Autodesk Inventor part; units mm, degrees
ref_plane "YZ Plane" through (0, 0, 0) normal (1, 0, 0) x (0, 1, 0)
ref_plane "XZ Plane" through (0, 0, 0) normal (0, 1, 0) x (-1, 0, 0)
ref_plane "XY Plane" through (0, 0, 0) normal (0, 0, 1) x (1, 0, 0)
sketch "Эскиз1" plane through (0, 0, 0) normal (0, 0, 1) x (1, 0, 0)
  line L0 (-90.9717, -10.4774) -> (94.0283, -10.4774)
  line L1 (94.0283, -10.4774) -> (94.0283, 19.5226)
  line L2 (94.0283, 19.5226) -> (-90.9717, 19.5226)
  line L3 (-90.9717, 19.5226) -> (-90.9717, -10.4774)
  dimension "d2" = 185
  dimension "parametr_D" = 30
extrude "Выдавливание1" add sketch "Эскиз1" along normal blind 180
fillet "Сопряжение1" radius 42 1 edges at (94.0283, 4.5226, 180)
sketch "Эскиз3" plane through (-90.9717, -10.4774, 0) normal (0, -1, 0) x (1, 0, 0)
  point P0 (115, 21.3555)
sketch "Эскиз4" plane through (-90.9717, -10.4774, 0) normal (0, -1, 0) x (1, 0, 0)
  point P0 (15, 33)
equation "\"d2\" = parametr_A_"
equation "\"parametr_D\" = parametr_C_"
equation "\"d4\" = parametr_B_"
properties part number "lw_6_part2"
The model under review builds one solid part; all positions refer to its coordinate system, in mm. Give positions to 0.01 mm unless a question says otherwise; leave off trailing zeros. Write each loop counter-clockwise with the first axis right and the second up, starting at its lowest first coordinate (ties: lowest second). Pieces come first, ordered by that corner, then holes.
1. For P1, Ø4, axis at x = 60, y = 10, coming from the +Z side; P2, Ø1, axis at x = 61.5, y = 2.5, coming from the +Z side; P3, Ø12, axis at x = -15, y = 1, coming from the -Z side, all flat-tipped, find the tip position at first contact; note any pin that passes through.
2. Wall thickness on L1, parallel to X at y = 14.75, z = 139.5; L2, parallel to X at y = 6.25, z = 151.5; L3, parallel to Z at x = 72.5, y = 9.75: over which ranges is each line inside the solid? List them lowest first.
3. Add section A-A, the plane z = 160. Write out the cut boundary in (x, y).
Worked answers:
1. P1: stops at z = 179.57
1. P2: stops at z = 179.03
1. P3: stops at z = 0
2. L1: x = -90.97 to 94
2. L2: x = -90.97 to 91.8
2. L3: z = 0 to 174.67
3. outline: (-90.97, -10.48) - (87.81, -10.48) - (87.81, 19.52) - (-90.97, 19.52) - close
